The model under review builds one solid part; all positions refer to its coordinate system, in mm. A direction names the side the tool comes from. Coordinates: 2 decimals unless noted, no trailing zeros. Write each loop counter-clockwise with the first axis right and the second up, starting at its lowest first coordinate (ties: lowest second). Pieces come first, ordered by that corner, then holes. Notation, with made-up numbers: M -35.75,8 L -10.75,8 A22 ccw -10.75,27 Z; hole C -34,19 d6. An arc over 180 degrees is marked long. Answer as CSV lines item,"result". Start each with the question number.
from build123d import *

# Parameters (mm, degrees)
SKETCH1_R           = 150
SKETCH1_R_2         = 125
BOSS_EXTRUDE1_DEPTH = 5
SKETCH2_R           = 150
SKETCH2_R_2         = 145
BOSS_EXTRUDE2_DEPTH = 300
SKETCH3_R           = 150
SKETCH3_R_2         = 125
BOSS_EXTRUDE3_DEPTH = 5
CUT_EXTRUDE1_REACH  = 152
SKETCH5_W           = 121
SKETCH5_H           = 76
CUT_EXTRUDE2_REACH  = 152
SKETCH7_R           = 1.6


with BuildPart() as part:
    # Sketch1 → Boss-Extrude1 (new body)
    with BuildSketch(Plane(origin=(0, 0, 0), x_dir=(1, 0, 0), z_dir=(0, 1, 0))):
        Circle(SKETCH1_R)
        Circle(SKETCH1_R_2, mode=Mode.SUBTRACT)
    extrude(amount=BOSS_EXTRUDE1_DEPTH)

    # Sketch2 → Boss-Extrude2 (add)
    with BuildSketch(Plane(origin=(0, 5, 0), x_dir=(1, 0, 0), z_dir=(0, 1, 0))):
        Circle(SKETCH2_R)
        Circle(SKETCH2_R_2, mode=Mode.SUBTRACT)
    extrude(amount=BOSS_EXTRUDE2_DEPTH)

    # Sketch3 → Boss-Extrude3 (add)
    with BuildSketch(Plane(origin=(0, 305, 0), x_dir=(1, 0, 0), z_dir=(0, 1, 0))):
        Circle(SKETCH3_R)
        Circle(SKETCH3_R_2, mode=Mode.SUBTRACT)
    extrude(amount=-BOSS_EXTRUDE3_DEPTH)

    # Sketch5 → Cut-Extrude1 (cut, up to next)
    with BuildSketch(Plane.XY, mode=Mode.PRIVATE) as cut_extrude1_sk1:
        with Locations((0, 228.75)):
            Rectangle(SKETCH5_W, SKETCH5_H)
    cut_extrude1_tool1 = extrude(cut_extrude1_sk1.sketch, amount=CUT_EXTRUDE1_REACH, mode=Mode.PRIVATE) & part.part
    add(cut_extrude1_tool1.solids().sort_by_distance((0, 228.75, 0))[0], mode=Mode.SUBTRACT)

    # Sketch7 → Cut-Extrude2 (cut, up to next)
    with BuildSketch(Plane.XY, mode=Mode.PRIVATE) as cut_extrude2_sk1:
        with Locations((56.95, 270.15)):
            Circle(SKETCH7_R)
    cut_extrude2_tool1 = extrude(cut_extrude2_sk1.sketch, amount=CUT_EXTRUDE2_REACH, mode=Mode.PRIVATE) & part.part
    add(cut_extrude2_tool1.solids().sort_by_distance((56.95, 270.15, 0))[0], mode=Mode.SUBTRACT)
    # Sketch7 → Cut-Extrude2 (cut, up to next)
    with BuildSketch(Plane.XY, mode=Mode.PRIVATE) as cut_extrude2_sk2:
        with Locations((56.95, 187.35)):
            Circle(SKETCH7_R)
    cut_extrude2_tool2 = extrude(cut_extrude2_sk2.sketch, amount=CUT_EXTRUDE2_REACH, mode=Mode.PRIVATE) & part.part
    add(cut_extrude2_tool2.solids().sort_by_distance((56.95, 187.35, 0))[0], mode=Mode.SUBTRACT)
    # Sketch7 → Cut-Extrude2 (cut, up to next)
    with BuildSketch(Plane.XY, mode=Mode.PRIVATE) as cut_extrude2_sk3:
        with Locations((-56.95, 270.15)):
            Circle(SKETCH7_R)
    cut_extrude2_tool3 = extrude(cut_extrude2_sk3.sketch, amount=CUT_EXTRUDE2_REACH, mode=Mode.PRIVATE) & part.part
    add(cut_extrude2_tool3.solids().sort_by_distance((-56.95, 270.15, 0))[0], mode=Mode.SUBTRACT)
    # Sketch7 → Cut-Extrude2 (cut, up to next)
    with BuildSketch(Plane.XY, mode=Mode.PRIVATE) as cut_extrude2_sk4:
        with Locations((-56.95, 187.35)):
            Circle(SKETCH7_R)
    cut_extrude2_tool4 = extrude(cut_extrude2_sk4.sketch, amount=CUT_EXTRUDE2_REACH, mode=Mode.PRIVATE) & part.part
    add(cut_extrude2_tool4.solids().sort_by_distance((-56.95, 187.35, 0))[0], mode=Mode.SUBTRACT)


solid = part.part
1) To check wall thickness, follow line 1 (Y direction, x = 56.95, z = 135); line 2 (Z direction, x = 0, y = 160). State the ranges of each line that lie inside material, in increasing order. Write a range as [from, to].
2) Tool access review of faces 4 (the flat face through (64, 5, -108)), 5 (the cylindrical face through (-124.88, 302.54, -5.5)): name each direction out of +Z, -Z, +X, -X, +Y, -Y from which nothing blocks a thin tool from reaching the whole face with its end or side.
3) Take a section at B-B on z = 0. Give the boundary of the cut face in (x, y).
4) Take a section at A-A on x = 0. Give the boundary of the cut face in (y, z), and give its area (3 significant figures).
5) Take a section at D-D on y = 199. Give the boundary of the cut face in (x, z).
6) Mouldability with a two-part tool opening along Z and no side actions: class faces 1 (the flat face through (-56, 0, -112)), 2 (the cylindrical face through (77.951, 150.435, -122.265)), 3 (the cylindrical face through (80.64, 150.36, -126.48)) as +Z half, -Z half, draft (parallel to the pull), parting line (faces both ways), or undercut.
7) Clearance check with flat-ended pins moving along their axes: pin 1 Ø5 at (x, y) = (-56.95, 187.35) entering from +Z; pin 2 Ø10 at (x, y) = (-64, 142) entering from -Z; pin 3 Ø4 at (x, y) = (-56.95, 270.15) entering from -Z. State where each tip first meets the part, or that it passes through.
8) Take a section at C-C on x = -108. Give the boundary of the cut face in (y, z), and give its area (3 significant figures).
Results:
1,line 1,"y = [0, 185.75], [188.95, 190.75], [266.75, 268.55], [271.75, 305]"
1,line 2,"z = [-150, -145], [145, 150]"
2,face 4,"none"
2,face 5,"+Y, -Y"
3,outline,"M -150,0 L -125,0 L -125,5 L -145,5 L -145,300 L -125,300 L -125,305 L -150,305 Z; M 125,0 L 150,0 L 150,305 L 125,305 L 125,300 L 145,300 L 145,5 L 125,5 Z"
4,outline,"M 0,-150 L 305,-150 L 305,-125 L 300,-125 L 300,-145 L 5,-145 L 5,-125 L 0,-125 Z; M 0,125 L 5,125 L 5,145 L 190.75,145 L 190.75,150 L 0,150 Z; M 266.75,145 L 300,145 L 300,125 L 305,125 L 305,150 L 266.75,150 Z"
4,area,"3,070 mm²"
5,outline,"M -60.5,131.78 L -60.5,137.26 A150 ccw long 60.5,137.26 L 60.5,131.78 A145 cw long Z"
6,face 1,"draft"
6,face 2,"undercut"
6,face 3,"parting line"
7,pin 1,"stops at z = 139.77"
7,pin 2,"stops at z = -137.91"
7,pin 3,"stops at z = -139.57"
8,outline,"M 0,-104.1 L 305,-104.1 L 305,-62.94 L 300,-62.94 L 300,-96.75 L 5,-96.75 L 5,-62.94 L 0,-62.94 Z; M 0,62.94 L 5,62.94 L 5,96.75 L 300,96.75 L 300,62.94 L 305,62.94 L 305,104.1 L 0,104.1 Z"
8,area,"5,160 mm²"
